from build123d import *

# Parameters (mm, degrees)
SKETCH_1_R      = 1.55
SKETCH_1_R_2    = 4.4
EXTRUDE_1_DEPTH = 1.2
FILLET_1_R      = 5


with BuildPart() as part:
    # 草图1 → 凸台-拉伸1 (new body)
    with BuildSketch(Plane(origin=(0, 0, 0), x_dir=(1, 0, 0), z_dir=(0, 1, 0))):
        with BuildLine():
            ThreePointArc((-7.5, 4.330127019), (0, 2.320508076), (7.5, 4.330127019))
            Line((7.5, 4.330127019), (131.842341019, 76.119211078))
            ThreePointArc((131.842341019, 76.119211078), (134.192561968, 79.234695458), (133.588070719, 83.090129515))
            ThreePointArc((133.588070719, 83.090129515), (0, 157.320508076), (-133.588070719, 83.090129515))
            ThreePointArc((-133.588070719, 83.090129515), (-134.192561968, 79.234695458), (-131.842341019, 76.119211078))
            Line((-131.842341019, 76.119211078), (-7.5, 4.330127019))
        make_face()
        with BuildLine():
            Line((-7.247844507, 12.26469459), (-6.434671709, 13.077867389))
            ThreePointArc((-6.434671709, 13.077867389), (-4.242640687, 13.077867389), (-4.242640687, 10.885836367))
            Line((-4.242640687, 10.885836367), (-5.055813485, 10.072663569))
            ThreePointArc((-5.055813485, 10.072663569), (-7.247844507, 10.072663569), (-7.247844507, 12.26469459))
        make_face(mode=Mode.SUBTRACT)
        with BuildLine():
            ThreePointArc((-44.398711306, 29.328649647), (-45.240569735, 32.470508076), (-42.098711306, 33.312366504))
            Line((-42.098711306, 33.312366504), (-17.85, 19.312366504))
            ThreePointArc((-17.85, 19.312366504), (-17.008141571, 16.170508076), (-20.15, 15.328649647))
            Line((-20.15, 15.328649647), (-44.398711306, 29.328649647))
        make_face(mode=Mode.SUBTRACT)
        with BuildLine():
            ThreePointArc((-8.485281374, 23.613758428), (-8.485281374, 25.80578945), (-6.293250353, 25.80578945))
            Line((-6.293250353, 25.80578945), (-4.772970773, 24.28550987))
            ThreePointArc((-4.772970773, 24.28550987), (-4.772970773, 22.093478849), (-6.965001795, 22.093478849))
            Line((-6.965001795, 22.093478849), (-8.485281374, 23.613758428))
        make_face(mode=Mode.SUBTRACT)
        with BuildLine():
            ThreePointArc((-76.441651246, 47.828649647), (-77.283509675, 50.970508076), (-74.141651246, 51.812366504))
            Line((-74.141651246, 51.812366504), (-49.89293994, 37.812366504))
            ThreePointArc((-49.89293994, 37.812366504), (-49.051081511, 34.670508076), (-52.19293994, 33.828649647))
            Line((-52.19293994, 33.828649647), (-76.441651246, 47.828649647))
        make_face(mode=Mode.SUBTRACT)
        with BuildLine():
            ThreePointArc((-108.484591186, 66.328649647), (-109.326449615, 69.470508076), (-106.184591186, 70.312366504))
            Line((-106.184591186, 70.312366504), (-81.93587988, 56.312366504))
            ThreePointArc((-81.93587988, 56.312366504), (-81.094021451, 53.170508076), (-84.23587988, 52.328649647))
            Line((-84.23587988, 52.328649647), (-108.484591186, 66.328649647))
        make_face(mode=Mode.SUBTRACT)
        with Locations(Location((-128.644111376, 80.623565294, 0), (0, 0, 270))):
            Circle(SKETCH_1_R, mode=Mode.SUBTRACT)
        with BuildLine():
            Line((6.965001795, 12.547537303), (8.485281374, 11.027257723))
            ThreePointArc((8.485281374, 11.027257723), (8.485281374, 8.835226701), (6.293250353, 8.835226701))
            Line((6.293250353, 8.835226701), (4.772970773, 10.355506281))
            ThreePointArc((4.772970773, 10.355506281), (4.772970773, 12.547537303), (6.965001795, 12.547537303))
        make_face(mode=Mode.SUBTRACT)
        with Locations(Location((0, 17.320508076, 0), (0, 0, 270))):
            Circle(SKETCH_1_R_2, mode=Mode.SUBTRACT)
        with BuildLine():
            ThreePointArc((6.434671709, 21.563148763), (4.242640687, 21.563148763), (4.242640687, 23.755179784))
            Line((4.242640687, 23.755179784), (5.055813485, 24.568352583))
            ThreePointArc((5.055813485, 24.568352583), (7.247844507, 24.568352583), (7.247844507, 22.376321561))
            Line((7.247844507, 22.376321561), (6.434671709, 21.563148763))
        make_face(mode=Mode.SUBTRACT)
        with BuildLine():
            Line((17.85, 19.312366504), (42.098711306, 33.312366504))
            ThreePointArc((42.098711306, 33.312366504), (45.240569735, 32.470508076), (44.398711306, 29.328649647))
            Line((44.398711306, 29.328649647), (20.15, 15.328649647))
            ThreePointArc((20.15, 15.328649647), (17.008141571, 16.170508076), (17.85, 19.312366504))
        make_face(mode=Mode.SUBTRACT)
        with BuildLine():
            Line((49.89293994, 37.812366504), (74.141651246, 51.812366504))
            ThreePointArc((74.141651246, 51.812366504), (77.283509675, 50.970508076), (76.441651246, 47.828649647))
            Line((76.441651246, 47.828649647), (52.19293994, 33.828649647))
            ThreePointArc((52.19293994, 33.828649647), (49.051081511, 34.670508076), (49.89293994, 37.812366504))
        make_face(mode=Mode.SUBTRACT)
        with BuildLine():
            Line((81.93587988, 56.312366504), (106.184591186, 70.312366504))
            ThreePointArc((106.184591186, 70.312366504), (109.326449615, 69.470508076), (108.484591186, 66.328649647))
            Line((108.484591186, 66.328649647), (84.23587988, 52.328649647))
            ThreePointArc((84.23587988, 52.328649647), (81.094021451, 53.170508076), (81.93587988, 56.312366504))
        make_face(mode=Mode.SUBTRACT)
        with Locations(Location((128.644111376, 80.623565294, 0), (0, 0, 270))):
            Circle(SKETCH_1_R, mode=Mode.SUBTRACT)
        with BuildLine():
            ThreePointArc((-121.36730718, 94.990040307), (-110.680666398, 107.251671759), (-98.761313169, 118.318781395))
            ThreePointArc((-98.761313169, 118.318781395), (-95.521742889, 118.026917726), (-95.813606558, 114.787347446))
            ThreePointArc((-95.813606558, 114.787347446), (-107.377205543, 104.050555333), (-117.74488457, 92.154894025))
            ThreePointArc((-117.74488457, 92.154894025), (-120.973669016, 91.761255861), (-121.36730718, 94.990040307))
        make_face(mode=Mode.SUBTRACT)
        with BuildLine():
            ThreePointArc((-90.69744613, 124.607801823), (-77.060254038, 133.472275238), (-62.564798823, 140.850193318))
            ThreePointArc((-62.564798823, 140.850193318), (-59.529158156, 139.681910073), (-60.697441401, 136.646269406))
            ThreePointArc((-60.697441401, 136.646269406), (-74.760254038, 129.48855838), (-87.990419937, 120.888660901))
            ThreePointArc((-87.990419937, 120.888660901), (-91.203503494, 121.394718266), (-90.69744613, 124.607801823))
        make_face(mode=Mode.SUBTRACT)
        with BuildLine():
            ThreePointArc((-53.086413848, 144.689196813), (-37.542339143, 149.478104688), (-21.580134422, 152.60219136))
            ThreePointArc((-21.580134422, 152.60219136), (-18.980744151, 150.646898487), (-20.936037023, 148.047508216))
            ThreePointArc((-20.936037023, 148.047508216), (-36.421821425, 145.016665454), (-51.501955642, 140.37069103))
            ThreePointArc((-51.501955642, 140.37069103), (-54.453437636, 141.737714818), (-53.086413848, 144.689196813))
        make_face(mode=Mode.SUBTRACT)
        with BuildLine():
            Line((-14.519984026, 21.084822608), (-116.100224104, 79.732201561))
            ThreePointArc((-116.100224104, 79.732201561), (-118.495458951, 83.044155809), (-117.619464681, 87.036501605))
            ThreePointArc((-117.619464681, 87.036501605), (-67.234108176, 129.958707986), (-3.090840664, 146.287859331))
            Line((-3.090840664, 146.287859331), (-5.5, 31.275793813))
            ThreePointArc((-5.5, 31.275793813), (-11.23227108, 27.262142065), (-14.519984026, 21.084822608))
        make_face(mode=Mode.SUBTRACT)
        with BuildLine():
            ThreePointArc((14.519984026, 21.084822608), (11.23227108, 27.262142065), (5.5, 31.275793813))
            Line((5.5, 31.275793813), (3.090840664, 146.287859331))
            ThreePointArc((3.090840664, 146.287859331), (67.234108176, 129.958707986), (117.619464681, 87.036501605))
            ThreePointArc((117.619464681, 87.036501605), (118.495458951, 83.044155809), (116.100224104, 79.732201561))
            Line((116.100224104, 79.732201561), (14.519984026, 21.084822608))
        make_face(mode=Mode.SUBTRACT)
        with BuildLine():
            ThreePointArc((95.813606558, 114.787347446), (95.521742889, 118.026917726), (98.761313169, 118.318781395))
            ThreePointArc((98.761313169, 118.318781395), (110.680666398, 107.251671759), (121.36730718, 94.990040307))
            ThreePointArc((121.36730718, 94.990040307), (120.973669016, 91.761255861), (117.74488457, 92.154894025))
            ThreePointArc((117.74488457, 92.154894025), (107.377205543, 104.050555333), (95.813606558, 114.787347446))
        make_face(mode=Mode.SUBTRACT)
        with Locations(Location((0, 151.820508076, 0), (0, 0, 270))):
            Circle(SKETCH_1_R, mode=Mode.SUBTRACT)
        with BuildLine():
            ThreePointArc((20.936037023, 148.047508216), (18.980744151, 150.646898487), (21.580134422, 152.60219136))
            ThreePointArc((21.580134422, 152.60219136), (37.542339143, 149.478104688), (53.086413848, 144.689196813))
            ThreePointArc((53.086413848, 144.689196813), (54.453437636, 141.737714818), (51.501955642, 140.37069103))
            ThreePointArc((51.501955642, 140.37069103), (36.421821425, 145.016665454), (20.936037023, 148.047508216))
        make_face(mode=Mode.SUBTRACT)
        with BuildLine():
            ThreePointArc((87.990419937, 120.888660901), (74.760254038, 129.48855838), (60.697441401, 136.646269406))
            ThreePointArc((60.697441401, 136.646269406), (59.529158156, 139.681910073), (62.564798823, 140.850193318))
            ThreePointArc((62.564798823, 140.850193318), (77.060254038, 133.472275238), (90.69744613, 124.607801823))
            ThreePointArc((90.69744613, 124.607801823), (91.203503494, 121.394718266), (87.990419937, 120.888660901))
        make_face(mode=Mode.SUBTRACT)
    extrude(amount=EXTRUDE_1_DEPTH)

    # 圆角1
    fillet_1_edges = [part.edges().sort_by_distance(p)[0] for p in [
        (3.090840664, 0.6, -146.287859331),
        (-3.090840664, 0.6, -146.287859331),
    ]]
    fillet(fillet_1_edges, radius=FILLET_1_R)


solid = part.part
Design review of the part built by this model. Coordinates are the model's own, in mm. A direction names the side the tool comes from. Coordinates: 2 decimals unless noted, no trailing zeros. Order: outer loops, then holes, each group sorted by start corner. A loop starts at its lowest first (then second) coordinate and runs counter-clockwise, first axis right, second up. Notation, with made-up numbers: (47, 37) -> (67, 37) arc R27 ccw to (67, 63) -> close; hole circle Ø2 at (-21.5, 34.5). An arc over 180 degrees is marked (long way). One line per item, written item: value.
1) Draft analysis for pull direction Z (two halves, no side actions). For faces 1 (the face through (74.95, 0.59, -129.38)), 2 (the face through (-1, 1.2, -86)), 3 (the face through (-64.15, 0.59, -40.73)), state which applies: +Z half, -Z half, draft (parallel to the pull), parting line (faces both ways), or undercut.
Output values:
face 1: undercut
face 2: draft
face 3: undercut
2) Machinability: for faces 4 (the face through (-1, 0, -86)), 5 (the face through (107.53, 0.59, -103.89)), which of the approach directions +Z, -Z, +X, -X, +Y, -Y give a long, thin tool a straight path to every point of the face, cutting with its end or side? Answer none if there is none.
Output values:
face 4: +Z, -Z, +X, -X, -Y
face 5: +Y, -Y
3) We need section C-C, the plane y = 0.55. Count the separate pieces of the cut face and the enclosed holes in it, then the cut area to 3 significant figures.
Output values:
separate pieces: 1
enclosed holes: 22
area: 6,000 mm2
4) We need section A-A, the plane z = -109. Give the boundary of the cut face in (x, y), then the cut area to 3 significant figures.
Output values:
outline: (-113.44, 0) -> (-108.96, 0) -> (-108.96, 1.2) -> (-113.44, 1.2) -> close; (-102.35, 0) -> (-97.62, 0) -> (-97.62, 1.2) -> (-102.35, 1.2) -> close; (-3.87, 0) -> (3.87, 0) -> (3.87, 1.2) -> (-3.87, 1.2) -> close; (97.62, 0) -> (102.35, 0) -> (102.35, 1.2) -> (97.62, 1.2) -> close; (108.96, 0) -> (113.44, 0) -> (113.44, 1.2) -> (108.96, 1.2) -> close
area: 31.4 mm2
5) To check wall thickness, follow probe 1 along X at (y, z) = (0.35, -43); probe 2 along Z at (x, y) = (82.5, 1); probe 3 along X at (y, z) = (1.15, -124). State the ranges of each line that lie inside material, in increasing order. Write a range as [from, to].
Output values:
probe 1: x = [-74.48, -68.08], [-58.88, -52.48], [-5.25, 5.25], [52.48, 58.88], [68.08, 74.48]
probe 2: z = [-133.95, -130.18], [-124.7, -120.84], [-60.33, -56.64], [-52.1, -47.63]
probe 3: x = [-96.82, -91.27], [-83.55, -77.68], [-3.56, 3.56], [77.68, 83.55], [91.27, 96.82]
6) We need section B-B, the plane z = -130.5. Give the boundary of the cut face in (x, y).
Output values:
outline: (-87.86, 0) -> (-81.99, 0) -> (-81.99, 1.2) -> (-87.86, 1.2) -> close; (-72.98, 0) -> (-66.18, 0) -> (-66.18, 1.2) -> (-72.98, 1.2) -> close; (-3.42, 0) -> (3.42, 0) -> (3.42, 1.2) -> (-3.42, 1.2) -> close; (66.18, 0) -> (72.98, 0) -> (72.98, 1.2) -> (66.18, 1.2) -> close; (81.99, 0) -> (87.86, 0) -> (87.86, 1.2) -> (81.99, 1.2) -> close
